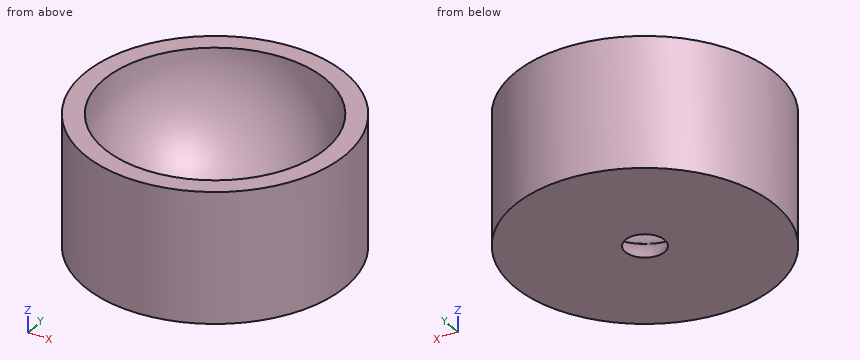
```python
from build123d import *

# Parameters (mm, degrees)
SKETCH1_R           = 10
BOSS_EXTRUDE1_DEPTH = 10
SKETCH3_R           = 1.5
CUT_EXTRUDE1_DEPTH  = 8
FILLET1_R           = 5


with BuildPart() as part:
    # Sketch1 → Boss-Extrude1 (new body)
    with BuildSketch(Plane.XY):
        Circle(SKETCH1_R)
    extrude(amount=BOSS_EXTRUDE1_DEPTH)

    # Sketch2 → Cut-Revolve1 (revolve, cut)
    with BuildSketch(Plane.XY.offset(10)):
        with BuildLine():
            Line((0, 8.5), (0, -8.5))
            ThreePointArc((0, -8.5), (8.5, 0), (0, 8.5))
        make_face()
    revolve(axis=Axis((0, 8.5, 10), (0, -1, 0)), mode=Mode.SUBTRACT)

    # Sketch3 → Cut-Extrude1 (cut)
    with BuildSketch(Plane(origin=(0, 0, 0), x_dir=(-1, 0, 0), z_dir=(0, 0, -1))):
        Circle(SKETCH3_R)
    extrude(amount=-CUT_EXTRUDE1_DEPTH, mode=Mode.SUBTRACT)

    # Fillet1
    # the kernel refuses this fillet: 5 mm, written as the material it takes off along each edge
    with BuildSketch(Plane(origin=(3e-09, 0, 1.633399735), x_dir=(-1, 0, 0), z_dir=(0, -1, 0))) as fillet1_piece_1:
        with BuildLine():
            CenterArc((6.052704826, 3.70049401), FILLET1_R, 204.419783659, 38.942441269)
            Line((3.810962297, -0.768800166), (3.766127446, -0.858186049))
            ThreePointArc((3.766127446, -0.858186049), (2.65159267, -0.396088594), (1.482352944, -0.098430591))
            Line((1.482352944, -0.098430591), (1.400000003, 0))
            ThreePointArc((1.400000003, 0), (1.399999997, 0.816699867), (1.408945901, 1.592057849))
            Line((1.408945901, 1.592057849), (1.499999997, 1.633399735))
        make_face()
    revolve(axis=Axis((3e-09, 0, 1.633399735), (0, 0, -1)), mode=Mode.SUBTRACT)


solid = part.part
```
Model file for the job. Use its own axes, mm. Round coordinates to 2 decimals unless told otherwise and drop trailing zeros. Write each loop counter-clockwise with the first axis right and the second up, starting at its lowest first coordinate (ties: lowest second). Pieces come first, ordered by that corner, then holes. Notation, with made-up numbers: (41.5, 56) -> (51.5, 56) arc R18 cw to (51.5, 71) -> close; hole circle Ø8 at (76.5, 89). An arc over 180 degrees is marked (long way). Answer as CSV lines item,"result".
1. Slice it at A-A, the plane y = 0. List the corners of the cut face in (x, z), plus the area to 3 significant figures.
Resolved:
outline,"(-10, 0) -> (-1.5, 0) arc R5 ccw to (-3.81, 2.4) arc R8.5 cw to (-8.5, 10) -> (-10, 10) -> close; (1.5, 0) -> (10, 0) -> (10, 10) -> (8.5, 10) arc R8.5 cw to (3.81, 2.4) arc R5 ccw to start"
area,"79.7 mm²"
2. Slice it at C-C, the plane z = 3.5. List the corners of the cut face in (x, y).
Resolved:
outline,"circle Ø20 at (0, 0); hole circle Ø10.95 at (0, 0)"
3. Pin check, flat tips, straight feed: pin 1 Ø1.5 at (x, z) = (-2.5, 8) entering from +Y; pin 2 Ø1 at (x, z) = (3.5, 3) entering from +Y; pin 3 Ø5 at (x, z) = (5, 7.5) entering from -Y. Stop position of each tip, or through.
Resolved:
pin 1,"y = 9.85"
pin 2,"y = 9.54"
pin 3,"y = -9.68"
4. Drill centre lines: line 1 (X direction, y = -5.5, z = 4.5); line 2 (Y direction, x = -3, z = 4.75); line 3 (Y direction, x = -4, z = 9.5). Where is each one in solid material? Low to high.
Resolved:
line 1,"-8.35 to -3.43, 3.43 to 8.35"
line 2,"-9.54 to -5.97, 5.97 to 9.54"
line 3,"-9.17 to -7.48, 7.48 to 9.17"
5. Slice it at D-D, the plane y = -8.25. List the corners of the cut face in (x, z).
Resolved:
outline,"(-5.65, 0) -> (5.65, 0) -> (5.65, 10) -> (2.05, 10) arc R2.05 cw to (-2.05, 10) -> (-5.65, 10) -> close"
6. Slice it at B-B, the plane x = -5.25. List the corners of the cut face in (y, z), plus the area to 3 significant figures.
Resolved:
outline,"(-8.51, 0) -> (8.51, 0) -> (8.51, 10) -> (6.68, 10) arc R6.68 cw to (-6.68, 10) -> (-8.51, 10) -> close"
area,"100 mm²"
